For this review, take the finished solid that the model builds, in its own axes (mm). Face numbers are marked on the shaded views. A direction names the side the tool comes from. Round coordinates to 2 decimals unless told otherwise and drop trailing zeros. Write each loop counter-clockwise with the first axis right and the second up, starting at its lowest first coordinate (ties: lowest second). Pieces come first, ordered by that corner, then holes. Notation, with made-up numbers: (26, -1.5) -> (41, -1.5) arc R15 ccw to (41, 16.5) -> close; hole circle Ø11 at (-9, 69). An arc over 180 degrees is marked (long way). Answer as CSV lines item,"result". Start each with the question number.
Item 1: For pin 1 Ø12.5 at (x, z) = (271, -21) entering from +Y; pin 2 Ø2.5 at (y, z) = (3, -9) entering from +X; pin 3 Ø5 at (x, y) = (210, 35.5) entering from -Z; pin 4 Ø10 at (x, y) = (142.5, 9) entering from -Z, all flat-tipped, find the tip position at first contact; note any pin that passes through.
Item 2: Mouldability with a two-part tool opening along Y and no side actions: class the marked faces 1, 2, 3 and 4 as +Y half, -Y half, draft (parallel to the pull), parting line (faces both ways), or undercut.
Item 3: Wall thickness on probe 1 along X at (y, z) = (31, -13); probe 2 along Y at (x, z) = (116.5, -19.5); probe 3 along Y at (x, z) = (-25, -31.75): over which ranges is each line inside the solid? List them lowest first. Write a range as from..to.
Item 4: Machinability: for the marked faces 5 and 6, which of the approach directions +Z, -Z, +X, -X, +Y, -Y give a long, thin tool a straight path to every point of the face, cutting with its end or side? Answer none if there is none.
Item 5: Take a section at A-A on x = 6.5. Give the boundary of the cut face in (y, z) (3 decimals), then the cut area to 3 significant figures.
Item 6: Take a section at B-B on y = 32.5. Give the boundary of the cut face in (x, z) (3 decimals).
```python
from build123d import *

# Parameters (mm, degrees)
BASE_FLANGE1_DEPTH           = 254
SKETCH6_W                    = 2.032
SKETCH6_H                    = 34.036
BOSS_EXTRUDE1_DEPTH          = 25.4
EDGE_FLANGE1_STRIP_W         = 14.478
EDGE_FLANGE1_STRIP_H         = 2.032
EDGE_FLANGE1_STRIP_CUT_DEPTH = 34.036
EDGE_FLANGE1_DEPTH           = 34.036
SKETCH10_R                   = 2.4511
CUT_EXTRUDE1_DEPTH           = 311.37147501
SKETCH11_R                   = 2.4511
CUT_EXTRUDE2_DEPTH           = 286.467638271
SKETCH12_R                   = 4.3688
CUT_EXTRUDE3_DEPTH           = 286.467638271
FILLET1_R                    = 3.175


# Sheet-metal steps are written as plain solids
with BuildPart() as part:
    # Sketch1 → Base-Flange1 (new body)
    with BuildSketch(Plane(origin=(0, 0, 0), x_dir=(0, 0, -1), z_dir=(1, 0, 0))):
        with BuildLine():
            Line((22.225, 0), (5.207, 0))
            ThreePointArc((5.207, 0), (1.52509499, 1.52509499), (0, 5.207))
            Line((0, 5.207), (0, 39.243))
            ThreePointArc((0, 39.243), (1.52509499, 42.92490501), (5.207, 44.45))
            Line((5.207, 44.45), (22.225, 44.45))
            Line((22.225, 44.45), (22.225, 42.418))
            Line((22.225, 42.418), (5.207, 42.418))
            ThreePointArc((5.207, 42.418), (2.96193597, 41.48806403), (2.032, 39.243))
            Line((2.032, 39.243), (2.032, 5.207))
            ThreePointArc((2.032, 5.207), (2.96193597, 2.96193597), (5.207, 2.032))
            Line((5.207, 2.032), (22.225, 2.032))
            Line((22.225, 2.032), (22.225, 0))
        make_face()
    extrude(amount=BASE_FLANGE1_DEPTH)

    # Sketch6 → Boss-Extrude1 (add)
    with BuildSketch(Plane(origin=(254, 0, 0), x_dir=(0, 0, -1), z_dir=(1, 0, 0))):
        with Locations((1.016, 22.225)):
            Rectangle(SKETCH6_W, SKETCH6_H)
    boss_extrude1 = extrude(amount=BOSS_EXTRUDE1_DEPTH)

    # Edge-Flange1 strip (across the edge) → Edge-Flange1 strip cut (cut)
    with BuildSketch(Plane(origin=(279.4, 39.243, -2.032), x_dir=(-1, 0, 0), z_dir=(0, -1, 0))):
        with Locations((-2.032, -1.016)):
            Rectangle(EDGE_FLANGE1_STRIP_W, EDGE_FLANGE1_STRIP_H)
    edge_flange1_strip_cut = extrude(amount=EDGE_FLANGE1_STRIP_CUT_DEPTH, mode=Mode.SUBTRACT)

    # Edge-Flange1 section (across the edge) → Edge-Flange1 (add)
    with BuildSketch(Plane(origin=(279.4, 39.243, -2.032), x_dir=(-1, 0, 0), z_dir=(0, -1, 0))):
        with BuildLine():
            Line((0, 3.175), (0, 36.068))
            Line((0, 36.068), (2.032, 36.068))
            Line((2.032, 36.068), (2.032, 3.175))
            ThreePointArc((2.032, 3.175), (2.96193597, 0.92993597), (5.207, 0))
            Line((5.207, 0), (5.207, -2.032))
            ThreePointArc((5.207, -2.032), (1.52509499, -0.50690501), (0, 3.175))
        make_face()
    edge_flange1 = extrude(amount=EDGE_FLANGE1_DEPTH)

    # Mirror1: Boss-Extrude1, Edge-Flange1 strip cut, Edge-Flange1 across plane
    add(boss_extrude1.mirror(Plane(origin=(127, 0, 0), x_dir=(0, 0, 1), z_dir=(1, 0, 0))))
    add(edge_flange1_strip_cut.mirror(Plane(origin=(127, 0, 0), x_dir=(0, 0, 1), z_dir=(1, 0, 0))), mode=Mode.SUBTRACT)
    add(edge_flange1.mirror(Plane(origin=(127, 0, 0), x_dir=(0, 0, 1), z_dir=(1, 0, 0))))

    # Sketch10 → Cut-Extrude1 (cut, through all)
    with BuildSketch(Plane(origin=(279.4, 0, 0), x_dir=(0, 0, -1), z_dir=(1, 0, 0))):
        with Locations((12.7, 22.225)):
            Circle(SKETCH10_R)
        with Locations((31.75, 22.225)):
            Circle(SKETCH10_R)
    extrude(amount=-CUT_EXTRUDE1_DEPTH, mode=Mode.SUBTRACT)

    # Sketch11 → Cut-Extrude2 (cut, through all)
    with BuildSketch(Plane(origin=(0, 44.45, 0), x_dir=(1, 0, 0), z_dir=(0, 1, 0))):
        with Locations(Location((12.7, 15.875, 0), (0, 0, 270))):
            Circle(SKETCH11_R)
        with Locations(Location((241.3, 15.875, 0), (0, 0, 270))):
            Circle(SKETCH11_R)
    extrude(amount=-CUT_EXTRUDE2_DEPTH, mode=Mode.SUBTRACT)

    # Sketch12 → Cut-Extrude3 (cut, through all)
    with BuildSketch(Plane.XY):
        with Locations((34.925, 22.225)):
            Circle(SKETCH12_R)
        with Locations((219.075, 22.225)):
            Circle(SKETCH12_R)
    extrude(amount=-CUT_EXTRUDE3_DEPTH, mode=Mode.SUBTRACT)

    # Fillet1
    fillet1_edges = [part.edges().sort_by_distance(p)[0] for p in [
        (-24.384, 5.207, -38.1),
        (0, 1.016, -22.225),
        (-24.384, 39.243, -38.1),
        (0, 43.434, -22.225),
        (254, 1.016, -22.225),
        (278.384, 39.243, -38.1),
        (278.384, 5.207, -38.1),
        (254, 43.434, -22.225),
    ]]
    fillet(fillet1_edges, radius=FILLET1_R)


solid = part.part
```
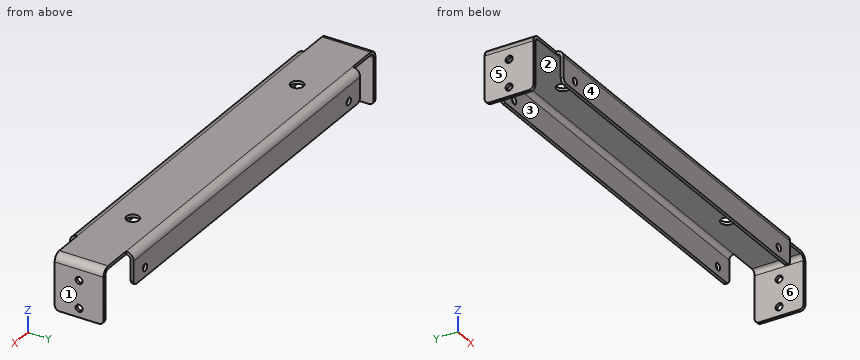
Output values:
1,pin 1,"passes through"
1,pin 2,"stops at x = 254"
1,pin 3,"stops at z = -2.03"
1,pin 4,"stops at z = -2.27"
2,face 1,"draft"
2,face 2,"undercut"
2,face 3,"undercut"
2,face 4,"-Y half"
3,probe 1,"x = -25.4..-23.37, 277.37..279.4"
3,probe 2,"y = 0..2.03, 42.42..44.45"
3,probe 3,"y = 5.21..19.77, 24.68..39.24"
4,face 5,"+Z, -Z, -X, +Y, -Y"
4,face 6,"-Z, +Y, -Y"
5,outline,"(0, -22.225) -> (2.032, -22.225) -> (2.032, -5.207) arc R3.175 cw to (5.207, -2.032) -> (39.243, -2.032) arc R3.175 cw to (42.418, -5.207) -> (42.418, -22.225) -> (44.45, -22.225) -> (44.45, -5.207) arc R5.207 ccw to (39.243, 0) -> (5.207, 0) arc R5.207 ccw to (0, -5.207) -> close"
5,area,"165 mm^2"
6,outline,"(-25.4, -38.1) -> (-23.368, -38.1) -> (-23.368, -5.207) arc R3.175 cw to (-20.193, -2.032) -> (274.193, -2.032) arc R3.175 cw to (277.368, -5.207) -> (277.368, -38.1) -> (279.4, -38.1) -> (279.4, -5.207) arc R5.207 ccw to (274.193, 0) -> (-20.193, 0) arc R5.207 ccw to (-25.4, -5.207) -> close"
